```python
from build123d import *

# Parameters (mm, degrees)
F0_R          = 85
F0_R_2        = 62.1020092735
F1_DEPTH      = 2.5
F2_R          = 85
F2_R_2        = 82.5
F3_DEPTH      = 25
F4_R          = 3
F5_DEPTH      = 85.001
F5_DEPTH_BACK = 85.001
F6_R          = 3
F7_DEPTH      = 85.0010001
F7_DEPTH_BACK = 85.0010001
F8_R          = 6
F9_DEPTH      = 25


with BuildPart() as f1:
    # F0 (on Front) → F1 (new body)
    with BuildSketch(Plane.XZ):
        Circle(F0_R)
        Circle(F0_R_2, mode=Mode.SUBTRACT)
    extrude(amount=F1_DEPTH)

    # F2 (on face) → F3 (join)
    with BuildSketch(Plane(origin=(0, 0, 0), x_dir=(-1, 0, 0), z_dir=(0, 1, 0))):
        Circle(F2_R)
        Circle(F2_R_2, mode=Mode.SUBTRACT)
    extrude(amount=F3_DEPTH)

    # F4 (on Top) → F5 (cut, two sides)
    with BuildSketch(Plane.XY) as f5_sk:
        with Locations((0, 7.5)):
            Circle(F4_R)
    extrude(amount=-F5_DEPTH, mode=Mode.SUBTRACT)
    extrude(f5_sk.sketch, amount=F5_DEPTH_BACK, mode=Mode.SUBTRACT)

    # F6 (on Right) → F7 (cut, two sides)
    with BuildSketch(Plane.YZ) as f7_sk:
        with Locations((7.5, 0)):
            Circle(F6_R)
    extrude(amount=F7_DEPTH, mode=Mode.SUBTRACT)
    extrude(f7_sk.sketch, amount=-F7_DEPTH_BACK, mode=Mode.SUBTRACT)

    # F8 (on Front) → F9 (cut)
    with BuildSketch(Plane.XZ):
        with Locations((42.4534804545, -63.6392331608)):
            Circle(F8_R)
    extrude(amount=F9_DEPTH, mode=Mode.SUBTRACT)


solid = f1.part
```
Geometry: final body of the model. Coordinates: model frame, mm. A direction names the side the tool comes from. Round coordinates to 2 decimals unless told otherwise and drop trailing zeros. Loops run counter-clockwise (first coordinate to the right, second up) from the corner with the lowest first, then second, coordinate; pieces in that order, holes last.
Item 1: Section A-A, the plane z = 0. Output: boundary loops of the cut face in (x, y), plus the area to 3 significant figures.
Checked values:
outline: (-85, -2.5) - (-62.1, -2.5) - (-62.1, 0) - (-82.5, 0) - (-82.5, 4.5) - (-85, 4.5) - close; (-85, 10.5) - (-82.5, 10.5) - (-82.5, 25) - (-85, 25) - close; (62.1, -2.5) - (85, -2.5) - (85, 4.5) - (82.5, 4.5) - (82.5, 0) - (62.1, 0) - close; (82.5, 10.5) - (85, 10.5) - (85, 25) - (82.5, 25) - close
area: 209 mm2
Item 2: Contact query for flat-ended pins moving along their axis: P1, Ø1, axis at y = 15.5, z = -42, coming from the +X side; P2, Ø12, axis at x = -29, y = 21, coming from the +Z side; P3, Ø5, axis at x = -63, z = -42, coming from the +Y side; P4, Ø5, axis at x = 0, y = 7.5, coming from the -Z side. Output: stop coordinate, or through.
Checked values:
P1: stops at x = 74.18
P2: stops at z = 81.83
P3: stops at y = 0
P4: passes through
Item 3: Section C-C, the plane x = 33. Output: boundary loops of the cut face in (y, z), plus the area to 3 significant figures.
Checked values:
outline: (-2.5, -78.33) - (25, -78.33) - (25, -75.61) - (0, -75.61) - (0, -52.61) - (-2.5, -52.61) - close; (-2.5, 52.61) - (0, 52.61) - (0, 75.61) - (25, 75.61) - (25, 78.33) - (-2.5, 78.33) - close
area: 265 mm2
Item 4: Line query: L1, parallel to Z at x = 0, y = 18.75; L2, parallel to Y at x = 23.5, z = 73.5. Output: solid intervals per line, ascending.
Checked values:
L1: z = -85 to -82.5, 82.5 to 85
L2: y = -2.5 to 0
Item 5: Section B-B, the plane x = 0. Output: boundary loops of the cut face in (y, z), plus the area to 3 significant figures.
Checked values:
outline: (-2.5, -85) - (4.5, -85) - (4.5, -82.5) - (0, -82.5) - (0, -62.1) - (-2.5, -62.1) - close; (-2.5, 62.1) - (0, 62.1) - (0, 82.5) - (4.5, 82.5) - (4.5, 85) - (-2.5, 85) - close; (10.5, -85) - (25, -85) - (25, -82.5) - (10.5, -82.5) - close; (10.5, 82.5) - (25, 82.5) - (25, 85) - (10.5, 85) - close
area: 209 mm2
Item 6: Section D-D, the plane y = 7.5. Output: boundary loops of the cut face in (x, z).
Checked values:
outline: (-84.95, -3) arc R85 ccw to (-3, -84.95) - (-3, -82.45) arc R82.5 cw to (-82.45, -3) - close; (-84.95, 3) - (-82.45, 3) arc R82.5 cw to (-3, 82.45) - (-3, 84.95) arc R85 ccw to start; (3, -84.95) arc R85 ccw to (84.95, -3) - (82.45, -3) arc R82.5 cw to (3, -82.45) - close; (3, 82.45) arc R82.5 cw to (82.45, 3) - (84.95, 3) arc R85 ccw to (3, 84.95) - close
Item 7: Mould query, pull axis Y, two halves, no side actions, for faces 3 (the flat face through (0, -2.5, 63)), 4 (the cylindrical face through (83.7, 10.27, -1.15)), 5 (the cylindrical face through (-3, 7.6, -83.7)), 6 (the flat face through (44, 25, 70)). Classes: released by +Y, released by -Y, zero draft, split by the parting line, or undercut.
Checked values:
face 3: released by -Y
face 4: undercut
face 5: undercut
face 6: released by +Y
Item 8: Reachability of faces 1 (the cylindrical face through (45.68, -1.23, -58.58)), 2 (the flat face through (-31, 0, -55)) from +Z, -Z, +X, -X, +Y, -Y: full face, straight path, thin tool, end or side. Return the list, or none.
Checked values:
face 1: +Y, -Y
face 2: +Y
